Read the model definition and answer for the solid it produces. Units are mm, in the model's axes. A direction names the side the tool comes from. Round coordinates to 2 decimals unless told otherwise and drop trailing zeros. Loops run counter-clockwise (first coordinate to the right, second up) from the corner with the lowest first, then second, coordinate; pieces in that order, holes last. Notation, with made-up numbers: (-38.75, -32) - (1.25, -32) arc R20 cw to (1.25, -20) - close; hole circle Ø6 at (-28.75, 14.5). An arc over 180 degrees is marked (long way). Use one line per item in the form item = value. Start each with the question number.
```python
from build123d import *

# Parameters (mm, degrees)
PAD045_DEPTH    = 5
SKETCH132_R     = 2.75
HOLE028_DEPTH   = 25
SKETCH141_R     = 5
PAD049_DEPTH    = 5
SKETCH136_R     = 2.8
POCKET041_DEPTH = 9.1


with BuildPart() as part:
    # Sketch129 → Pad045 (new body)
    with BuildSketch(Plane.XY):
        with BuildLine():
            ThreePointArc((-9.213418, 97.472873), (0, 95.5), (9.213418, 97.472873))
            Line((9.213418, 97.472873), (60.634406, 46.051885))
            ThreePointArc((60.634406, 46.051885), (71.94812, 46.05189), (71.948104, 57.365604))
            Line((20.527127, 108.786582), (71.948104, 57.365604))
            ThreePointArc((20.527127, 108.786582), (22.5, 118), (20.527127, 127.213418))
            Line((20.527127, 127.213418), (71.948104, 178.634396))
            ThreePointArc((71.948104, 178.634396), (71.948104, 189.948104), (60.634396, 189.948104))
            Line((9.213418, 138.527127), (60.634396, 189.948104))
            ThreePointArc((9.213418, 138.527127), (0, 140.5), (-9.213418, 138.527127))
            Line((-9.213418, 138.527127), (-60.634396, 189.948104))
            ThreePointArc((-60.634396, 189.948104), (-71.948104, 189.948104), (-71.948104, 178.634396))
            Line((-20.527127, 127.213418), (-71.948104, 178.634396))
            ThreePointArc((-20.527127, 127.213418), (-22.5, 118), (-20.527127, 108.786582))
            Line((-20.527127, 108.786582), (-71.948121, 57.365588))
            ThreePointArc((-71.948121, 57.365588), (-71.948112, 46.051882), (-60.634406, 46.051885))
            Line((-9.213418, 97.472873), (-60.634406, 46.051885))
        make_face()
    extrude(amount=PAD045_DEPTH)

    # Sketch132 → Hole028 (cut)
    with BuildSketch(Plane.XY.offset(6)):
        with Locations((10, 128)):
            Circle(SKETCH132_R)
        with Locations((10, 108)):
            Circle(SKETCH132_R)
        with Locations((-10, 108)):
            Circle(SKETCH132_R)
        with Locations((-10, 128)):
            Circle(SKETCH132_R)
    extrude(amount=-HOLE028_DEPTH, mode=Mode.SUBTRACT)

    # Sketch141 (on Face5 of Hole028) → Pad049 (join)
    with BuildSketch(Plane.XY.offset(5)):
        with Locations((-66.291261, 51.708739)):
            Circle(SKETCH141_R)
        with Locations((66.291261, 51.708739)):
            Circle(SKETCH141_R)
        with Locations((66.291261, 184.291261)):
            Circle(SKETCH141_R)
        with Locations((-66.291261, 184.291261)):
            Circle(SKETCH141_R)
    extrude(amount=PAD049_DEPTH)

    # Sketch136 (on Face30 of Pad049) → Pocket041 (cut)
    with BuildSketch(Plane.XY.offset(10)):
        with Locations((-66.291261, 184.291261)):
            Circle(SKETCH136_R)
        with Locations((66.291261, 184.291261)):
            Circle(SKETCH136_R)
        with Locations((66.291261, 51.708739)):
            Circle(SKETCH136_R)
        with Locations((-66.291261, 51.708739)):
            Circle(SKETCH136_R)
    extrude(amount=-POCKET041_DEPTH, mode=Mode.SUBTRACT)


with BuildPart() as part_1:
    # Body020 placement: moved
    add(part.part.moved(Location((0, 0, 10))))


solid = part_1.part
```
1) A cutting plane is placed at A-A on z = 17.25. Write down the section's boundary in (x, y), plus the area to 3 significant figures.
2) Flat-ended cylindrical pins translate along their axes: pin 1 (4 mm diameter, centred on y = 74.5, z = 12.5, fed in from +X); pin 2 (1 mm diameter, centred on x = -1, y = 138, fed in from +Z); pin 3 (5 mm diameter, centred on x = -29, z = 11.5, fed in from +Y). Find the tip coordinate at first contact, or state that the pin passes through.
3) Straight lines are drawn through the part: line 1 (Y direction, x = 10, z = 12.1); line 2 (Y direction, x = 64, z = 16.5); line 3 (X direction, y = 128, z = 12.5). For each, find the intervals that lie inside material, in ascending order. Write a range as from..to.
4) A cutting plane is placed at C-C on y = 84.5. Write down the section's boundary in (x, z), plus the area to 3 significant figures.
5) A cutting plane is placed at B-B on x = 38. Write down the section's boundary in (y, z), plus the area to 3 significant figures.
6) For faces 5 (the flat face through (34.564, 72.122, 12.465)), 6 (the cylindrical face through (65.68, 181.56, 15.51)), 7 (the flat face through (-34.564, 163.878, 12.465)), determine the directions among +Z, -Z, +X, -X, +Y, -Y from which every point of the face is accessible in a straight line to the end or side of a thin tool.
7) A cutting plane is placed at D-D on y = 113. Write down the section's boundary in (x, z), plus the area to 3 significant figures.
8) Determine the mould class of faces 1 (the flat face through (45.878, 152.564, 12.465)), 2 (the flat face through (-34.564, 72.122, 12.465)), 3 (the flat face through (68.4, 49.6, 20)), 4 (the flat face through (-45.878, 83.436, 12.465)) for opening direction X: +X half, -X half, draft (parallel to the pull), parting line (faces both ways), or undercut.
Checks:
q1.outline = circle Ø10 at (-66.29, 51.71); circle Ø10 at (-66.29, 184.29); circle Ø10 at (66.29, 51.71); circle Ø10 at (66.29, 184.29); hole circle Ø5.6 at (-66.29, 51.71); hole circle Ø5.6 at (-66.29, 184.29); hole circle Ø5.6 at (66.29, 51.71); hole circle Ø5.6 at (66.29, 184.29)
q1.area = 216 mm²
q2.pin_1 = 56.81
q2.pin_2 = 15
q2.pin_3 = 160.81
q3.line_1 = 96.69..105.25, 110.75..125.25, 130.75..139.31
q3.line_2 = 47.26..50.1, 53.32..56.15, 179.85..182.68, 185.9..188.74
q3.line_3 = -21.31..-12.75, -7.25..7.25, 12.75..21.31
q4.outline = (-44.81, 10) - (-22.19, 10) - (-22.19, 15) - (-44.81, 15) - close; (22.19, 10) - (44.81, 10) - (44.81, 15) - (22.19, 15) - close
q4.area = 226 mm²
q5.outline = (68.69, 10) - (91.31, 10) - (91.31, 15) - (68.69, 15) - close; (144.69, 10) - (167.31, 10) - (167.31, 15) - (144.69, 15) - close
q5.area = 226 mm²
q6.face_5 = +Z, -Z, -Y
q6.face_6 = +Z
q6.face_7 = +Z, -Z, +Y
q7.outline = (-21.94, 10) - (21.94, 10) - (21.94, 15) - (-21.94, 15) - close
q7.area = 219 mm²
q8.face_1 = +X half
q8.face_2 = undercut
q8.face_3 = draft
q8.face_4 = -X half
